```python
from build123d import *

# Parameters (mm, degrees)
BOSS_EXTRUDE1_DEPTH                              = 6
SKETCH2_W                                        = 26
SKETCH2_H                                        = 11
CBORE_FOR_M4_HEX_HEAD_MACHINE_SCREW1_D           = 4.5
CBORE_FOR_M4_HEX_HEAD_MACHINE_SCREW1_DEPTH       = 32
CBORE_FOR_M4_HEX_HEAD_MACHINE_SCREW1_CBORE_D     = 7.5
CBORE_FOR_M4_HEX_HEAD_MACHINE_SCREW1_CBORE_DEPTH = 4.1
F_12_0_12_DIAMETER_HOLE1_D                       = 12
FILLET1_R                                        = 0.375
FILLET2_R                                        = 0.625


with BuildPart() as part:
    # Sketch1 → Boss-Extrude1 (new body)
    with BuildSketch(Plane(origin=(0, 0, 0), x_dir=(0, -1, 0), z_dir=(-1, 0, 0))):
        with BuildLine():
            Line((-1.696016468, 20.93140053), (-20.93140053, 1.696016468))
            ThreePointArc((-20.93140053, 1.696016468), (-21, 0), (-20.93140053, -1.696016468))
            Line((-20.93140053, -1.696016468), (-1.696016468, -20.93140053))
            ThreePointArc((-1.696016468, -20.93140053), (0, -21), (1.696016468, -20.93140053))
            Line((1.696016468, -20.93140053), (20.93140053, -1.696016468))
            ThreePointArc((20.93140053, -1.696016468), (21, 0), (20.93140053, 1.696016468))
            Line((20.93140053, 1.696016468), (1.696016468, 20.93140053))
            ThreePointArc((1.696016468, 20.93140053), (0, 21), (-1.696016468, 20.93140053))
        make_face()
    extrude(amount=-BOSS_EXTRUDE1_DEPTH)

    # Sketch2 → Revolve1 (revolve)
    with BuildSketch(Plane.XY, mode=Mode.PRIVATE) as revolve1_sk:
        with Locations((19, 5.5)):
            Rectangle(SKETCH2_W, SKETCH2_H)
    revolve(revolve1_sk.sketch.rotate(Axis((6, 0, 0), (1, 0, 0)), 270), axis=Axis((6, 0, 0), (1, 0, 0)))

    # CBORE for M4 Hex Head Machine Screw1
    with Locations(Plane.ZY):
        with Locations((0, 16), (0, -16), (-16, 0), (16, 0)):
            CounterBoreHole(CBORE_FOR_M4_HEX_HEAD_MACHINE_SCREW1_D / 2, CBORE_FOR_M4_HEX_HEAD_MACHINE_SCREW1_CBORE_D / 2, CBORE_FOR_M4_HEX_HEAD_MACHINE_SCREW1_CBORE_DEPTH, depth=CBORE_FOR_M4_HEX_HEAD_MACHINE_SCREW1_DEPTH)

    # Ø12.0 (12) Diameter Hole1 (through all)
    with Locations(Plane.ZY):
        with Locations((0, 0)):
            Hole(F_12_0_12_DIAMETER_HOLE1_D / 2)

    # Fillet1
    fillet1_edges = [part.edges().sort_by_distance(p)[0] for p in [
        (0, 21, 0),
        (0, 0, 21),
        (6, 21, 0),
        (6, 0, -21),
        (6, -21, 0),
        (6, 0, 21),
        (0, -21, 0),
        (0, 0, -21),
    ]]
    fillet(fillet1_edges, radius=FILLET1_R)

    # Fillet2
    fillet2_edges = [part.edges().sort_by_distance(p)[0] for p in [
        (32, 0, 11),
        (0, 0, 6),
        (32, 0, 6),
    ]]
    fillet(fillet2_edges, radius=FILLET2_R)


solid = part.part
```
Here's how the part is built. I have some questions about the finished solid (model axes, mm). A direction names the side the tool comes from. Give positions to 0.01 mm unless a question says otherwise; leave off trailing zeros. Loops run counter-clockwise (first coordinate to the right, second up) from the corner with the lowest first, then second, coordinate; pieces in that order, holes last. Notation, with made-up numbers: M -17,63 L 1,63 A16 ccw 1,73 Z; hole C 76.5,-18 d4. An arc over 180 degrees is marked long. Return JSON: item names as keys, results as strings.
Item 1: Please list where these lines run through material, in increasing order: line 1 (Y direction, x = 2.45, z = 16); line 2 (Y direction, x = 5, z = -16); line 3 (X direction, y = -6, z = 2.5).
A:
{"line 1": "y = -6.63 to -3.75, 3.75 to 6.63", "line 2": "y = -6.63 to -2.25, 2.25 to 6.63", "line 3": "x = 0.01 to 31.99"}
Item 2: Thinking about a two-plate mould opening in Y: for faces 4 (the flat face through (2.96, 11.18, 11.45)), 5 (the flat face through (2.96, -11.18, -11.45)), 6 (the cylindrical face through (2.02, 12.34, -0.81)), which applies, released by +Y, released by -Y, zero draft, split by the parting line, or undercut?
A:
{"face 4": "released by +Y", "face 5": "released by -Y", "face 6": "undercut"}
Item 3: On a 3-axis mill with a long thin cutter (end or side, diameter ignored), from which of +Z, -Z, +X, -X, +Y, -Y can I reach the whole of each face in a straight line? I mean faces 1 (the cylindrical face through (5.063, 0.676, 13.854)), 2 (the cylindrical face through (2.021, 0.165, -19.746)), 3 (the flat face through (6, 6.2, 9.3)). Say none if no direction works.
A:
{"face 1": "+X, -X", "face 2": "-X", "face 3": "+X"}
Item 4: Imagine slicing it at B-B on z = 0. State how many separate pieces and enclosed holes the cut face has, then the cut area to 3 significant figures.
A:
{"separate pieces": "4", "enclosed holes": "0", "area": "361 mm^2"}
Item 5: I'm going to push flat-ended pins straight in: pin 1 Ø2 at (y, z) = (1.5, 16) entering from -X; pin 2 Ø1 at (y, z) = (-14, 5) entering from +X; pin 3 Ø4 at (x, z) = (16, -3.5) entering from +Y. Where does each tip first touch, or does it pass through?
A:
{"pin 1": "stops at x = 4.1", "pin 2": "stops at x = 6", "pin 3": "stops at y = 10.9"}
Item 6: Imagine slicing it at A-A on x = 5. List the corners of the cut face in (y, z) for me.
A:
{"outline": "M -20.93,-1.7 L -1.7,-20.93 A21 ccw 1.7,-20.93 L 20.93,-1.7 A21 ccw 20.93,1.7 L 1.7,20.93 A21 ccw -1.7,20.93 L -20.93,1.7 A21 ccw Z; hole C -16,0 d4.5; hole C 0,0 d12; hole C 0,-16 d4.5; hole C 0,16 d4.5; hole C 16,0 d4.5"}
Item 7: Imagine slicing it at D-D on y = -16. List the corners of the cut face in (x, z) for me.
A:
{"outline": "M 0,-6.63 L 6,-6.63 L 6,-2.25 L 4.1,-2.25 L 4.1,-3.75 L 0,-3.75 Z; M 0,3.75 L 4.1,3.75 L 4.1,2.25 L 6,2.25 L 6,6.63 L 0,6.63 Z"}
